Geometry: final body of the model. Coordinates: model frame, mm. Face numbers are marked on the shaded views. A direction names the side the tool comes from. Round coordinates to 2 decimals unless told otherwise and drop trailing zeros. Order: outer loops, then holes, each group sorted by start corner. A loop starts at its lowest first (then second) coordinate and runs counter-clockwise, first axis right, second up. Notation, with made-up numbers: M -20.75,32.5 L 5.25,32.5 A15 ccw 5.25,59.5 Z; hole C 16,31 d11. An arc over 180 degrees is marked long. Put each result on its own line as item: value. Start each with the question number.
1) Section B-B, the plane x = 0. Return loops of the section in (y, z).
2) Material intervals for probe 1 along Y at (x, z) = (0, 6.3); probe 2 along Y at (x, z) = (-1, 2); probe 3 along Y at (x, z) = (-15, 2.8), sorted ascending. Write a range as [from, to].
3) Access query for the marked faces 1, 2 and 3. Directions: +Z, -Z, +X, -X, +Y, -Y. A direction counts if a zero-diameter tool reaches every point of the face in a straight line with its end or side. Return the directions, or none.
4) Section A-A, the plane z = 2. Return loops of the section in (x, y).
5) Section C-C, the plane y = 0. Count the separate pieces of the cut face and the enclosed holes in it, then the cut area to 3 significant figures.
6) First-contact query: P1, Ø3, axis at x = -0.5, y = -2, coming from the +Z side; P2, Ø6, axis at y = -4.5, z = 7.5, coming from the +X side; P3, Ø3, axis at x = 15, y = 0, coming from the -Z side; P4, Ø2, axis at y = 19, z = 2.5, coming from the +X side. Flat tips, straight axial feed; report the tip coordinate or a pass-through.
7) Draft query along X for the marked faces 4, 5 and 6. Return one class per face: pulls with the +X half, pulls with the -X half, needs draft (parallel to the pull), parting line crosses it, or undercut.
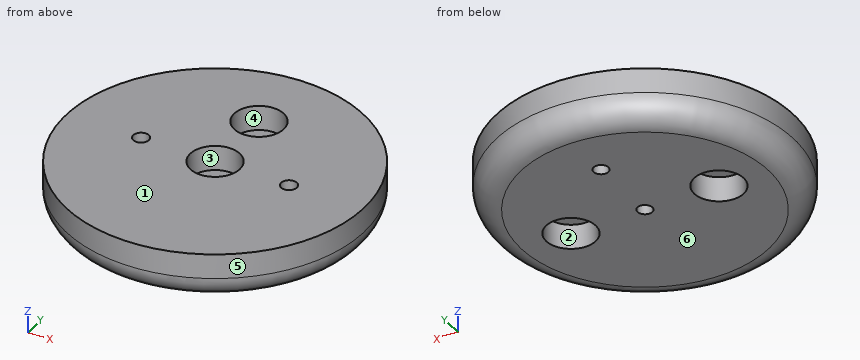
from build123d import *

# Parameters (mm, degrees)
SKETCH_R        = 30
PAD_DEPTH       = 10
SKETCH002_R     = 1.5
POCKET_DEPTH    = 10.001
SKETCH003_R     = 5
POCKET001_DEPTH = 5
SKETCH004_R     = 1.6
POCKET002_DEPTH = 10.001
SKETCH005_R     = 5
POCKET003_DEPTH = 5
FILLET_R        = 5


with BuildPart() as part:
    # Sketch → Pad (new body)
    with BuildSketch(Plane.XY):
        Circle(SKETCH_R)
    extrude(amount=PAD_DEPTH)

    # Sketch002 (on Face3 of Pad) → Pocket (cut, through all)
    with BuildSketch(Plane.XY.offset(10)):
        Circle(SKETCH002_R)
        with Locations((0, 15)):
            Circle(SKETCH002_R)
    extrude(amount=-POCKET_DEPTH, mode=Mode.SUBTRACT)

    # Sketch003 (on Face3 of Pocket) → Pocket001 (cut)
    with BuildSketch(Plane.XY.offset(10)):
        with Locations((0, 15)):
            Circle(SKETCH003_R)
        Circle(SKETCH003_R)
    extrude(amount=-POCKET001_DEPTH, mode=Mode.SUBTRACT)

    # Sketch004 (on Face2 of Pocket001) → Pocket002 (cut, through all)
    with BuildSketch(Plane(origin=(0, 0, 0), x_dir=(1, 0, 0), z_dir=(0, 0, -1))):
        with Locations((-15, 0)):
            Circle(SKETCH004_R)
        with Locations((15, 0)):
            Circle(SKETCH004_R)
    extrude(amount=-POCKET002_DEPTH, mode=Mode.SUBTRACT)

    # Sketch005 (on Face2 of Pocket002) → Pocket003 (cut)
    with BuildSketch(Plane(origin=(0, 0, 0), x_dir=(1, 0, 0), z_dir=(0, 0, -1))):
        with Locations((-15, 0)):
            Circle(SKETCH005_R)
        with Locations((15, 0)):
            Circle(SKETCH005_R)
    extrude(amount=-POCKET003_DEPTH, mode=Mode.SUBTRACT)

    # Fillet
    fillet_edges = [part.edges().sort_by_distance(p)[0] for p in [
        (-30, 0, 0),
    ]]
    fillet(fillet_edges, radius=FILLET_R)


solid = part.part
Result sheet:
1. outline: M -30,5 A5 ccw -25,0 L -1.5,0 L -1.5,5 L -5,5 L -5,10 L -30,10 Z; M 1.5,0 L 13.5,0 L 13.5,5 L 10,5 L 10,10 L 5,10 L 5,5 L 1.5,5 Z; M 16.5,0 L 25,0 A5 ccw 30,5 L 30,10 L 20,10 L 20,5 L 16.5,5 Z
2. probe 1: y = [-30, -5], [5, 10], [20, 30]
2. probe 2: y = [-28.98, -1.12], [1.12, 13.88], [16.12, 28.98]
2. probe 3: y = [-25.39, -5], [5, 25.39]
3. face 1: +Z, +X, -X, +Y, -Y
3. face 2: -Z
3. face 3: +Z
4. outline: C 0,0 d58; hole C -15,0 d10; hole C 0,0 d3; hole C 0,15 d3; hole C 15,0 d10
5. separate pieces: 4
5. enclosed holes: 0
5. area: 392 mm2
6. P1: stops at z = 5
6. P2: stops at x = 29.96
6. P3: passes through
6. P4: stops at x = 23.38
7. face 4: undercut
7. face 5: parting line crosses it
7. face 6: needs draft
